For this review, take the finished solid that the model builds, in its own axes (mm). Face numbers are marked on the shaded views. A direction names the side the tool comes from. Give positions to 0.01 mm unless a question says otherwise; leave off trailing zeros. Write each loop counter-clockwise with the first axis right and the second up, starting at its lowest first coordinate (ties: lowest second). Pieces come first, ordered by that corner, then holes. Notation, with made-up numbers: (24, 12) -> (67, 12) arc R22 ccw to (67, 44) -> close; hole circle Ø9 at (47, 58). An arc over 180 degrees is marked (long way). Write item = value, one per line.
Autodesk Inventor part; units mm, degrees
ref_plane "YZ Plane" through (0, 0, 0) normal (1, 0, 0) x (0, 1, 0)
ref_plane "XZ Plane" through (0, 0, 0) normal (0, 1, 0) x (-1, 0, 0)
ref_plane "XY Plane" through (0, 0, 0) normal (0, 0, 1) x (1, 0, 0)
sketch "Esboço1" plane through (0, 0, 0) normal (0, 0, 1) x (1, 0, 0)
  line L0 (-33.417, 5) -> (-95.5408, 55.4046)
  line L1 (-95.5408, 55.4046) -> (-118.417, 46.6482)
  line L2 (-118.417, 46.6482) -> (-120.5199, 35.1357)
  line L3 (-120.5199, 35.1357) -> (-97.358, 44.0015)
  line L4 (-97.358, 44.0015) -> (-22.0526, -17.098)
  line L5 (0, 0) -> (-33.417, 0)
  line L6 (-33.417, 5) -> (6.583, 5)
  line L7 (6.583, 5) -> (6.583, 0)
  line L8 (6.583, 0) -> (-33.417, 0)
  line L9 (-33.417, 0) -> (-33.417, 5)
  line L10 (-33.417, -5) -> (-95.5408, -55.4046)
  line L11 (-95.5408, -55.4046) -> (-118.417, -46.6482)
  line L12 (-118.417, -46.6482) -> (-120.5199, -35.1357)
  line L13 (-120.5199, -35.1357) -> (-97.358, -44.0015)
  line L14 (-97.358, -44.0015) -> (-22.0526, 17.098)
  line L15 (-33.417, -5) -> (6.583, -5)
  line L16 (6.583, -5) -> (6.583, 0)
  line L17 (-33.417, 0) -> (-33.417, -5)
  point P0 (-43.126, 0)
  dimension "d2" = 10
  dimension "d4" = 120
  dimension "d7" = 10
  dimension "d8" = 80
  dimension "d10" = 40
  dimension "d11" = 5
  dimension "d12" = 125
  dimension "d13" = 35.1357
extrude "Extrusão1" add sketch "Esboço1" along normal blind 20
properties part number "pinca"
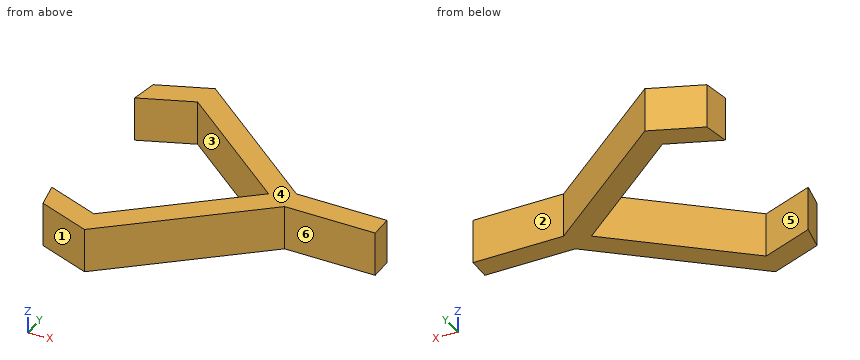
(1) Take a section at C-C (x = -53). Write out the cut boundary in (y, z).
Answers below:
outline = (-20.89, 0) -> (-8.01, 0) -> (-8.01, 20) -> (-20.89, 20) -> close; (8.01, 0) -> (20.89, 0) -> (20.89, 20) -> (8.01, 20) -> close
(2) Tool access review of the marked faces 1, 2 and 3: name each direction out of +Z, -Z, +X, -X, +Y, -Y from which nothing blocks a thin tool from reaching the whole face with its end or side.
Answers below:
face_1 = +Z, -Z, -X, -Y
face_2 = +Z, -Z, +X, +Y
face_3 = +Z, -Z
(3) The part is to be moulded in two halves that separate along Y. For the marked faces 4, 5 and 6, say which applies: released by +Y, released by -Y, zero draft, split by the parting line, or undercut.
Answers below:
face_4 = zero draft
face_5 = undercut
face_6 = released by -Y
(4) For pin 1 (8 mm diameter, centred on x = -67.5, y = 39.5, fed in from +Z); pin 2 (6 mm diameter, centred on y = 38.5, z = 13.5, fed in from -X); pin 3 (1 mm diameter, centred on y = -19, z = 8, fed in from -X); pin 4 (12 mm diameter, centred on x = -21.5, z = 5, fed in from -Y), all flat-tipped, find the tip position at first contact; note any pin that passes through.
Answers below:
pin_1 = through
pin_2 = -120.45
pin_3 = -67.16
pin_4 = -5
(5) To check wall thickness, follow probe 1 along Y at (x, z) = (-7, 5.25); probe 2 along Y at (x, z) = (-86, 2.5); probe 3 along Y at (x, z) = (-79, 10). State the ranges of each line that lie inside material, in increasing order.
Answers below:
probe_1 = -5 to 5
probe_2 = -47.66 to -34.79, 34.79 to 47.66
probe_3 = -41.98 to -29.11, 29.11 to 41.98
(6) Take a section at D-D (y = 23). Write out the cut boundary in (x, z).
Answers below:
outline = (-71.47, 0) -> (-55.6, 0) -> (-55.6, 20) -> (-71.47, 20) -> close
(7) Take a section at A-A (x = -90). Write out the cut boundary in (y, z).
Answers below:
outline = (-50.91, 0) -> (-38.03, 0) -> (-38.03, 20) -> (-50.91, 20) -> close; (38.03, 0) -> (50.91, 0) -> (50.91, 20) -> (38.03, 20) -> close
(8) Take a section at B-B (z = 9.5). Write out the cut boundary in (x, y).
Answers below:
outline = (-120.52, -35.14) -> (-118.42, -46.65) -> (-95.54, -55.4) -> (-33.42, -5) -> (6.58, -5) -> (6.58, 5) -> (-33.42, 5) -> (-95.54, 55.4) -> (-118.42, 46.65) -> (-120.52, 35.14) -> (-97.36, 44) -> (-43.13, 0) -> (-97.36, -44) -> close
